```python
from build123d import *

# Parameters (mm, degrees)
F1_DEPTH = 50
F3_DEPTH = 50
F4_R     = 2


with BuildPart() as f1:
    # F0 (on Right) → F1 (new body)
    with BuildSketch(Plane.YZ):
        with BuildLine():
            Line((-27.136585, 14.208124), (-20, 14.208124))
            ThreePointArc((-20, 14.208124), (-20.068162, 39.737556), (-10, 63.197919))
            Line((-10, 63.197919), (-15.019473, 68.217392))
            ThreePointArc((-15.019473, 68.217392), (-26.643162, 42.461309), (-27.136585, 14.208124))
        make_face()
    extrude(amount=F1_DEPTH)

    # F2 (on Front) → F3 (cut)
    with BuildSketch(Plane.XZ):
        with BuildLine():
            Line((6.021636, 22.501509), (6.021636, 21.914739))
            ThreePointArc((6.021636, 21.914739), (8.147091, 20.21354), (10, 22.208124))
            ThreePointArc((10, 22.208124), (8.147091, 24.202708), (6.021636, 22.501509))
        make_face()
        with BuildLine():
            ThreePointArc((6.021636, 22.501509), (6, 22.208124), (6.021636, 21.914739))
            Line((6.021636, 21.914739), (6.021636, 22.501509))
        make_face()
        with BuildLine():
            ThreePointArc((6.021636, 22.501509), (8.147091, 24.202708), (10, 22.208124))
            Line((10, 22.208124), (10, 30.208124))
            ThreePointArc((10, 30.208124), (8.147091, 28.21354), (6.021636, 29.914739))
            Line((6.021636, 29.914739), (6.021636, 22.501509))
        make_face()
        with BuildLine():
            ThreePointArc((6.021636, 29.914739), (8.147091, 28.21354), (10, 30.208124))
            ThreePointArc((10, 30.208124), (7.852909, 32.202708), (6.021636, 29.914739))
        make_face()
        with BuildLine():
            ThreePointArc((40, 22.208124), (42, 20.208124), (44, 22.208124))
            ThreePointArc((44, 22.208124), (42, 24.208124), (40, 22.208124))
        make_face()
        with BuildLine():
            ThreePointArc((40, 22.208124), (42, 24.208124), (44, 22.208124))
            Line((44, 22.208124), (44, 30.208124))
            ThreePointArc((44, 30.208124), (42, 28.208124), (40, 30.208124))
            Line((40, 30.208124), (40, 22.208124))
        make_face()
        with BuildLine():
            ThreePointArc((40, 30.208124), (42, 28.208124), (44, 30.208124))
            ThreePointArc((44, 30.208124), (42, 32.208124), (40, 30.208124))
        make_face()
    extrude(amount=F3_DEPTH, mode=Mode.SUBTRACT)

    # F4
    f4_edges = [f1.edges().sort_by_distance(p)[0] for p in [
        (50, -23.568293, 14.208124),
        (50, -20.068162, 39.737556),
        (50, -12.509737, 65.707655),
        (50, -26.643162, 42.461309),
        (25, -10, 63.197919),
        (25, -15.019473, 68.217392),
        (0, -12.509737, 65.707655),
        (0, -23.568293, 14.208124),
        (0, -20.068162, 39.737556),
        (0, -26.643162, 42.461309),
        (25, -27.136585, 14.208124),
        (25, -20, 14.208124),
    ]]
    fillet(f4_edges, radius=F4_R)


solid = f1.part
```
Could you check a few things on this model? Use its own coordinates, in mm. A direction names the side the tool comes from. Coordinates: 2 decimals unless noted, no trailing zeros. Order: outer loops, then holes, each group sorted by start corner. A loop starts at its lowest first (then second) coordinate and runs counter-clockwise, first axis right, second up. Notation, with made-up numbers: M 62,-23 L 69,-23 A23 cw 69,11 Z; hole C 36.5,-38.5 d8. An arc over 180 degrees is marked long. Use one line per item in the form item = value. Start each with the question number.
1. Please list where these lines run through material, in increasing order: line 1 (X direction, y = -22.75, z = 30.5); line 2 (X direction, y = -22, z = 28.5); line 3 (Y direction, x = 3, z = 28).
2. Suppose I cut it at B-B on x = 32.5. Write out the boundary of the cut face in (y, z), then the cut area to 3 significant figures.
3. Suppose I cut it at A-A on x = 8. Write out the boundary of the cut face in (y, z).
4. On a 3-axis mill with a long thin cutter (end or side, diameter ignored), from which of +Z, -Z, +X, -X, +Y, -Y can I reach the whole of each face in a straight line? I mean faces 5 (the cylindrical face through (49.43, -12.69, 65.04)), 6 (the flat face through (44, -25, 26)). Say none if no direction works.
5. We'd pull the mould along Z, two halves only. Please class faces 1 (the cylindrical face through (41.96, -24.51, 20.21)), 2 (the cylindrical face through (24.68, -26.64, 42.47)), 3 (the flat face through (40, -25, 26)), 4 (the cylindrical face through (49.4, -23.91, 14.78)): +Z half, -Z half, draft (parallel to the pull), parting line (faces both ways), or undercut.
6. For pin 1 (3 mm diameter, centred on x = 15, y = -17, fed in from +Z); pin 2 (3 mm diameter, centred on x = 14, z = 42.5, fed in from +Y); pin 3 (10 mm diameter, centred on x = 11, z = 60.5, fed in from -Y), each with a flat end and sliding along its axis, tell me the tip position at first contact or that it passes through.
Geometry says:
q1.line_1 = 0.06 to 6.02, 9.98 to 40.02, 43.98 to 49.94
q1.line_2 = 0.5 to 6.02, 10 to 40, 44 to 49.5
q1.line_3 = -28.34 to -21.34
q2.outline = M -27.43,15.89 A2 ccw -25.46,14.21 L -22.42,14.21 A2 ccw -20.44,16.54 A63 cw -10.91,61.85 A2 ccw -11.17,64.37 L -13.33,66.53 A2 ccw -16.41,66.23 A70 ccw Z
q2.area = 375 mm^2
q3.outline = M -28.16,32.21 L -21.14,32.21 A63 cw -10.91,61.85 A2 ccw -11.17,64.37 L -13.33,66.53 A2 ccw -16.41,66.23 A70 ccw Z; M -28,20.21 A70 ccw -27.43,15.89 A2 ccw -25.46,14.21 L -22.42,14.21 A2 ccw -20.44,16.54 A63 cw -20.96,20.21 Z
q4.face_5 = +Z, +X, +Y
q4.face_6 = +Y, -Y
q5.face_1 = undercut
q5.face_2 = parting line
q5.face_3 = undercut
q5.face_4 = -Z half
q6.pin_1 = 66.97
q6.pin_2 = -19.04
q6.pin_3 = -22.34
